Input: part model. Units: mm. Frame: model coordinates. A direction names the side the tool comes from. Coordinates: 2 decimals unless noted, no trailing zeros. Loops run counter-clockwise (first coordinate to the right, second up) from the corner with the lowest first, then second, coordinate; pieces in that order, holes last.
Autodesk Inventor part; units mm, degrees
ref_plane "YZ Plane" through (0, 0, 0) normal (1, 0, 0) x (0, 1, 0)
ref_plane "XZ Plane" through (0, 0, 0) normal (0, 1, 0) x (-1, 0, 0)
ref_plane "XY Plane" through (0, 0, 0) normal (0, 0, 1) x (1, 0, 0)
sketch "Sketch1" plane through (0, 0, 0) normal (0, 1, 0) x (-1, 0, 0)
  line L0 (99, 99) -> (-99, 99)
  line L1 (-99, 99) -> (-99, -99)
  line L2 (-99, -99) -> (99, -99)
  line L3 (99, -99) -> (99, 99)
  line L4 (99, 99) -> (-99, -99) construction
  line L5 (-99, 99) -> (99, -99) construction
  point P0 (0, 0)
  dimension "d0" = 198
  dimension "d1" = 198
extrude "Box" add sketch "Sketch1" along normal blind 198
sketch "Sketch2" plane through (99, 0, 99) normal (1, 0, 0) x (0, 0, -1)
  point P0 (99, 0)
  point P1 (99, 99)
hole "DecAxisHole" at (99, 99, 0) direction (-1, 0, 0) diameter 66 depth 198
sketch "Sketch3" plane through (0, 0, 0) normal (0, -1, 0) x (1, 0, 0)
  point P0 (0, 0)
  point P1 (-76, -76)
  point P2 (76, -76)
  point P3 (76, 76)
  point P4 (-76, 76)
hole "BoltHoles" at (-76, 0, -76) at (76, 0, -76) at (76, 0, 76) at (-76, 0, 76) direction (0, 1, 0) diameter 8 depth 24 tip angle 118
properties part number "RaDecConnector"
Item 1: Line query: L1, parallel to X at y = 12.25, z = 76; L2, parallel to Y at x = 24.5, z = 0. Output: solid intervals per line, ascending.
Result:
L1: x = -99 to -80, -72 to 72, 80 to 99
L2: y = 0 to 66, 132 to 198
Item 2: Reachability of faces 1 (the face through (-99, 54, -1)), 2 (the face through (79.905, 12.168, 76.867)) from +Z, -Z, +X, -X, +Y, -Y: full face, straight path, thin tool, end or side. Return the list, or none.
Result:
face 1: +Z, -Z, -X, +Y, -Y
face 2: -Y
Item 3: Section query A-A (z = 0). Output: boundary loops of the cut face in (x, y), then the cut area to 3 significant figures.
Result:
outline: (-99, 0) - (99, 0) - (99, 66) - (-99, 66) - close; (-99, 132) - (99, 132) - (99, 198) - (-99, 198) - close
area: 26,100 mm2
Item 4: Mould query, pull axis X, two halves, no side actions, for faces 3 (the face through (-76.678, 25.986, 76.151)), 4 (the face through (99, 54, 1)), 5 (the face through (-1.386, 128.277, -15.227)). Classes: +X half, -X half, draft (parallel to the pull), parting line (faces both ways), or undercut.
Result:
face 3: undercut
face 4: +X half
face 5: draft
Item 5: Contact query for flat-ended pins moving along their axis: P1, Ø6.5, axis at x = -76, z = 76, coming from the -Y side; P2, Ø7, axis at x = 76, z = -76, coming from the -Y side. Output: stop coordinate, or through.
Result:
P1: stops at y = 24.45
P2: stops at y = 24.3
Item 6: Section query B-B (x = -29.5). Output: boundary loops of the cut face in (y, z).
Result:
outline: (0, -99) - (198, -99) - (198, 99) - (0, 99) - close; hole circle Ø66 at (99, 0)
